Part model, mm, in its own coordinate system. A direction names the side the tool comes from. Coordinates: 2 decimals unless noted, no trailing zeros. Write each loop counter-clockwise with the first axis right and the second up, starting at its lowest first coordinate (ties: lowest second). Pieces come first, ordered by that corner, then holes. Notation, with made-up numbers: (69.25, -15) - (128.25, -15) arc R21 cw to (128.25, 7) - close; hole circle Ø11 at (-10, 73). An arc over 180 degrees is marked (long way). Use a Markdown table: item, result.
```python
from build123d import *

# Parameters (mm, degrees)
CROQUIS1_R              = 46
CROQUIS1_R_2            = 4
SALIENTE_EXTRUIR1_DEPTH = 4
CROQUIS2_R              = 50
CROQUIS2_R_2            = 46
SALIENTE_EXTRUIR2_DEPTH = 80
CORTAR_EXTRUIR1_DEPTH   = 10
CROQUIS4_R              = 54
CROQUIS4_R_2            = 50
CORTAR_EXTRUIR2_DEPTH   = 3


with BuildPart() as part:
    # Croquis1 → Saliente-Extruir1 (new body)
    with BuildSketch(Plane(origin=(0, 0, 0), x_dir=(0, 0, -1), z_dir=(1, 0, 0))):
        with BuildLine():
            Line((-49, 59), (49, 59))
            ThreePointArc((49, 59), (56.071067812, 56.071067812), (59, 49))
            Line((59, 49), (59, -49))
            ThreePointArc((59, -49), (56.071067812, -56.071067812), (49, -59))
            Line((49, -59), (-49, -59))
            ThreePointArc((-49, -59), (-56.071067812, -56.071067812), (-59, -49))
            Line((-59, -49), (-59, 49))
            ThreePointArc((-59, 49), (-56.071067812, 56.071067812), (-49, 59))
        make_face()
        Circle(CROQUIS1_R, mode=Mode.SUBTRACT)
        with Locations((45, -45)):
            Circle(CROQUIS1_R_2, mode=Mode.SUBTRACT)
        with Locations((-45, -45)):
            Circle(CROQUIS1_R_2, mode=Mode.SUBTRACT)
        with Locations((-45, 45)):
            Circle(CROQUIS1_R_2, mode=Mode.SUBTRACT)
        with Locations((45, 45)):
            Circle(CROQUIS1_R_2, mode=Mode.SUBTRACT)
    extrude(amount=SALIENTE_EXTRUIR1_DEPTH)

    # Croquis2 → Saliente-Extruir2 (add)
    with BuildSketch(Plane(origin=(4, 0, 0), x_dir=(0, 0, -1), z_dir=(1, 0, 0))):
        Circle(CROQUIS2_R)
        Circle(CROQUIS2_R_2, mode=Mode.SUBTRACT)
    extrude(amount=SALIENTE_EXTRUIR2_DEPTH)

    # Croquis3 → Cortar-Extruir1 (cut)
    with BuildSketch(Plane.XY.offset(50)):
        with BuildLine():
            Line((84, 0), (84, 4))
            Line((84, 4), (38, 4))
            ThreePointArc((38, 4), (34, 0), (38, -4))
            Line((38, -4), (84, -4))
            Line((84, -4), (84, 0))
        make_face()
    extrude(amount=-CORTAR_EXTRUIR1_DEPTH, mode=Mode.SUBTRACT)

    # Croquis4 → Cortar-Extruir2 (cut)
    with BuildSketch(Plane.ZY):
        Circle(CROQUIS4_R)
        with Locations(Location((0, 0, 0), (0, 0, 355.411434264))):
            Circle(CROQUIS4_R_2, mode=Mode.SUBTRACT)
    extrude(amount=-CORTAR_EXTRUIR2_DEPTH, mode=Mode.SUBTRACT)


solid = part.part
```
Item 1: Band-saw the part on A-A, the plane z = 0. Give the cut face in (x, y), then the cut area to 3 significant figures.
From the geometry:
| item | result |
|---|---|
| outline | (0, -59) - (4, -59) - (4, -50) - (84, -50) - (84, -46) - (0, -46) - (0, -50) - (3, -50) - (3, -54) - (0, -54) - close; (0, 46) - (84, 46) - (84, 50) - (4, 50) - (4, 59) - (0, 59) - (0, 54) - (3, 54) - (3, 50) - (0, 50) - close |
| area | 720 mm^2 |
Item 2: Band-saw the part on C-C, the plane z = 43. Give the cut face in (x, y).
From the geometry:
| item | result |
|---|---|
| outline | (0, -59) - (4, -59) - (4, -48.46) - (0, -48.46) - close; (0, -41.54) - (4, -41.54) - (4, -25.51) - (84, -25.51) - (84, -16.34) - (0, -16.34) - (0, -25.51) - (3, -25.51) - (3, -32.66) - (0, -32.66) - close; (0, 16.34) - (84, 16.34) - (84, 25.51) - (4, 25.51) - (4, 41.54) - (0, 41.54) - (0, 32.66) - (3, 32.66) - (3, 25.51) - (0, 25.51) - close; (0, 48.46) - (4, 48.46) - (4, 59) - (0, 59) - close |
Item 3: Drop flat-ended pins along their axis: P1, Ø10.5, axis at y = -45, z = 45, coming from the +X side; P2, Ø6, axis at x = 30.5, z = -26, coming from the -Y side; P3, Ø12, axis at x = 55.5, y = 21, coming from the -Z side; P4, Ø12, axis at y = 39.5, z = -13, coming from the +X side. Give the stop position or say it passes through.
From the geometry:
| item | result |
|---|---|
| P1 | x = 4 |
| P2 | y = -44.4 |
| P3 | z = -47.7 |
| P4 | x = 84 |
Item 4: Band-saw the part on D-D, the plane z = -42.5. Give the cut face in (x, y), then the cut area to 3 significant figures.
From the geometry:
| item | result |
|---|---|
| outline | (0, -59) - (4, -59) - (4, -48.12) - (0, -48.12) - close; (0, -41.88) - (4, -41.88) - (4, -26.34) - (84, -26.34) - (84, -17.6) - (0, -17.6) - (0, -26.34) - (3, -26.34) - (3, -33.31) - (0, -33.31) - close; (0, 17.6) - (84, 17.6) - (84, 26.34) - (4, 26.34) - (4, 41.88) - (0, 41.88) - (0, 33.31) - (3, 33.31) - (3, 26.34) - (0, 26.34) - close; (0, 48.12) - (4, 48.12) - (4, 59) - (0, 59) - close |
| area | 1,640 mm^2 |
Item 5: Which spindle directions (+Z, -Z, +X, -X, +Y, -Y) get a long thin tool onto all of the face, cutting with end or side? Do faces 1 (the face through (2, -59, -1)), 2 (the face through (1.479, -47.787, -14.709)), 3 (the face through (4, 1, 52)), 4 (the face through (41.412, 13.817, -43.876)), 5 (the face through (34, 0, 48)). Say none if no direction does.
From the geometry:
| item | result |
|---|---|
| face 1 | +Z, -Z, +X, -X, -Y |
| face 2 | -X |
| face 3 | +X |
| face 4 | +X, -X |
| face 5 | +Z, +X |
Item 6: Drill centre lines: probe 1 along Y at (x, z) = (1, 0); probe 2 along Y at (x, z) = (53, 0). Where is each one in solid material? Low to high.
From the geometry:
| item | result |
|---|---|
| probe 1 | -59 to -54, -50 to -46, 46 to 50, 54 to 59 |
| probe 2 | -50 to -46, 46 to 50 |
Item 7: Two-plate mould, pull along Z, no slides. Class faces 6 (the face through (1.972, -41.034, -44.479)), 7 (the face through (1.97, 55.99, 56.15)), 8 (the face through (61, -4, 48)): pulls with the +Z half, pulls with the -Z half, needs draft (parallel to the pull), parting line crosses it, or undercut.
From the geometry:
| item | result |
|---|---|
| face 6 | undercut |
| face 7 | pulls with the +Z half |
| face 8 | needs draft |
Item 8: Band-saw the part on B-B, the plane y = 0. Give the cut face in (x, z).
From the geometry:
| item | result |
|---|---|
| outline | (0, -59) - (4, -59) - (4, -50) - (84, -50) - (84, -46) - (0, -46) - (0, -50) - (3, -50) - (3, -54) - (0, -54) - close; (0, 46) - (34, 46) - (34, 50) - (4, 50) - (4, 59) - (0, 59) - (0, 54) - (3, 54) - (3, 50) - (0, 50) - close |
